Source: three-view drawing plus pictorial views. Frame: mm from the lowest corner of the part. A direction names the side the tool comes from. Give positions to 0.01 mm unless a question says otherwise; leave off trailing zeros. Write each loop counter-clockwise with the first axis right and the second up, starting at its lowest first coordinate (ties: lowest second). Pieces come first, ordered by that corner, then holes.
Q1. Draft query along X for the marked faces 3, 4 and 5. Return one class per face: pulls with the +X half, pulls with the -X half, needs draft (parallel to the pull), parting line crosses it, or undercut.
Q2. Reachability of the marked faces 1 and 2 from +Z, -Z, +X, -X, +Y, -Y: full face, straight path, thin tool, end or side. Return the list, or none.
Q3. Cut plane B-B on z = 125. Return the cut outline in (x, y).
Q4. Cut plane A-A on x = 125. Return the cut outline in (y, z).
Q5. Cut plane C-C on x = 44. Return the cut outline in (y, z), plus the area to 3 significant figures.
Q6. Cut plane D-D on z = 210. Return the cut outline in (x, y), plus the area to 3 significant figures.
Q7. Pin query (flat end, axial travel): pin 1 (1 mm diameter, centred on x = 54, y = 5, fed in from -Z); pin 2 (25 mm diameter, centred on x = 125, z = 35, fed in from +Y); pin 3 (8 mm diameter, centred on x = 222, y = 3, fed in from -Z). Return the tip coordinate at first contact, or that it passes through.
Q8. Line query: L1, parallel to Z at x = 125, y = 18.3; L2, parallel to Y at x = 128, z = 65.5; L3, parallel to Z at x = 125, y = 10. Output: solid intervals per line, ascending.
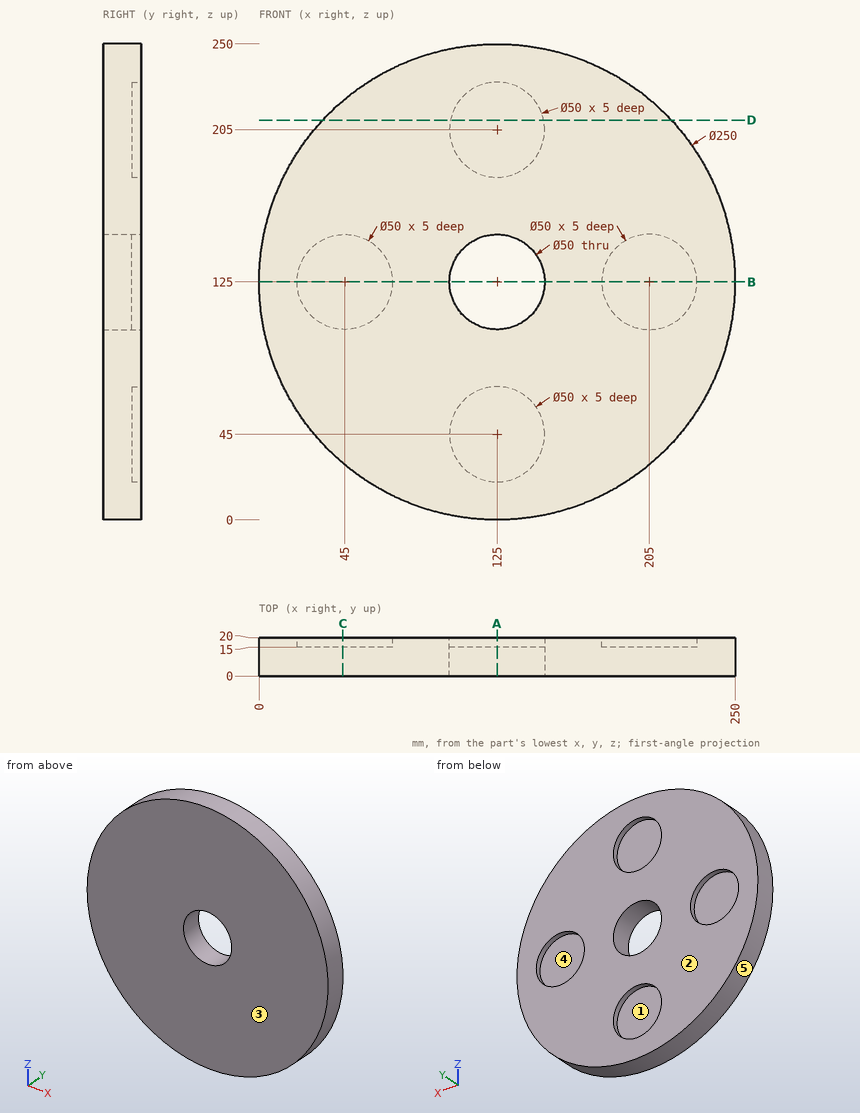
Data:
1. face 3: needs draft
1. face 4: undercut
1. face 5: parting line crosses it
2. face 1: +Y
2. face 2: +Z, -Z, +X, -X, +Y
3. outline: (0, 0) - (100, 0) - (100, 20) - (70, 20) - (70, 15) - (20, 15) - (20, 20) - (0, 20) - close; (150, 0) - (250, 0) - (250, 20) - (230, 20) - (230, 15) - (180, 15) - (180, 20) - (150, 20) - close
4. outline: (0, 0) - (20, 0) - (20, 20) - (15, 20) - (15, 70) - (20, 70) - (20, 100) - (0, 100) - close; (0, 150) - (20, 150) - (20, 180) - (15, 180) - (15, 230) - (20, 230) - (20, 250) - (0, 250) - close
5. outline: (0, 29.79) - (20, 29.79) - (20, 100.02) - (15, 100.02) - (15, 149.98) - (20, 149.98) - (20, 220.21) - (0, 220.21) - close
5. area: 3,560 mm2
6. outline: (33.35, 0) - (216.65, 0) - (216.65, 20) - (149.49, 20) - (149.49, 15) - (100.51, 15) - (100.51, 20) - (33.35, 20) - close
6. area: 3,420 mm2
7. pin 1: stops at z = 21.78
7. pin 2: stops at y = 15
7. pin 3: stops at z = 41.48
8. L1: z = 0 to 20, 70 to 100, 150 to 180, 230 to 250
8. L2: y = 0 to 15
8. L3: z = 0 to 100, 150 to 250
